from build123d import *

# Parameters (mm, degrees)
SKETCH1_W           = 50.8
SKETCH1_H           = 40.64
SKETCH1_R           = 2.0193
BOSS_EXTRUDE1_DEPTH = 1.5875


with BuildPart() as part:
    # Sketch1 → Boss-Extrude1 (new body, symmetric)
    with BuildSketch(Plane(origin=(0, 0, 0), x_dir=(1, 0, 0), z_dir=(0, 1, 0))):
        Rectangle(SKETCH1_W, SKETCH1_H)
        with Locations((-15.875, 12.7)):
            Circle(SKETCH1_R, mode=Mode.SUBTRACT)
        with Locations((15.875, 12.7)):
            Circle(SKETCH1_R, mode=Mode.SUBTRACT)
        with Locations((15.875, -12.7)):
            Circle(SKETCH1_R, mode=Mode.SUBTRACT)
        with Locations((-15.875, -12.7)):
            Circle(SKETCH1_R, mode=Mode.SUBTRACT)
    extrude(amount=BOSS_EXTRUDE1_DEPTH, both=True)


solid = part.part
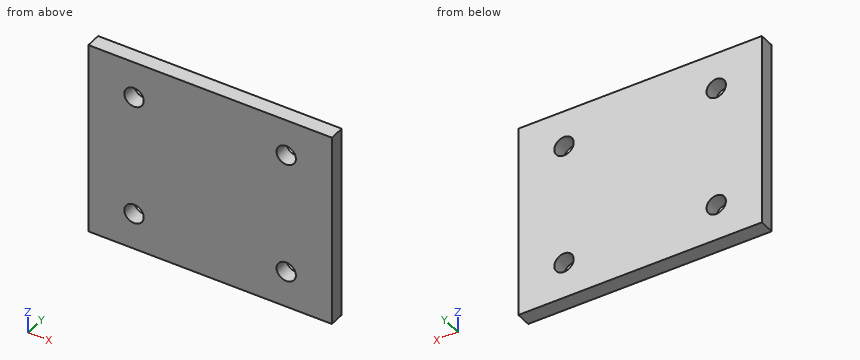
The model under review builds one solid part; all positions refer to its coordinate system, in mm. Round coordinates to 2 decimals unless told otherwise and drop trailing zeros. Loops run counter-clockwise (first coordinate to the right, second up) from the corner with the lowest first, then second, coordinate; pieces in that order, holes last. Notation, with made-up numbers: (28.25, 63) -> (54.25, 63) arc R7 cw to (54.25, 73) -> close; hole circle Ø5 at (72.5, -20). An arc over 180 degrees is marked (long way). Return JSON: item names as keys, results as strings.
(1) Add section A-A on y = 1.05. Write out the cut boundary in (x, z) (3 decimals).
Solved:
{"outline": "(-25.4, -20.32) -> (25.4, -20.32) -> (25.4, 20.32) -> (-25.4, 20.32) -> close; hole circle Ø4.039 at (-15.875, -12.7); hole circle Ø4.039 at (-15.875, 12.7); hole circle Ø4.039 at (15.875, -12.7); hole circle Ø4.039 at (15.875, 12.7)"}
(2) For line 1 (X direction, y = 0.75, z = -12.7); line 2 (X direction, y = -1.45, z = 12), list the stretches that pass through material, from the lowest coordinate up.
Solved:
{"line 1": "-25.4 to -17.89, -13.86 to 13.86, 17.89 to 25.4", "line 2": "-25.4 to -17.77, -13.98 to 13.98, 17.77 to 25.4"}
(3) Add section B-B on z = -12.7. Write out the cut boundary in (x, y), plus the area to 3 significant figures.
Solved:
{"outline": "(-25.4, -1.59) -> (-17.89, -1.59) -> (-17.89, 1.59) -> (-25.4, 1.59) -> close; (-13.86, -1.59) -> (13.86, -1.59) -> (13.86, 1.59) -> (-13.86, 1.59) -> close; (17.89, -1.59) -> (25.4, -1.59) -> (25.4, 1.59) -> (17.89, 1.59) -> close", "area": "136 mm2"}
